The model under review builds one solid part; all positions refer to its coordinate system, in mm. A direction names the side the tool comes from. Coordinates: 2 decimals unless noted, no trailing zeros. Loops run counter-clockwise (first coordinate to the right, second up) from the corner with the lowest first, then second, coordinate; pieces in that order, holes last. Notation, with made-up numbers: M -12,14 L 3,14 A21 ccw 3,45 Z; hole C 39.5,-0.5 d11. An arc over 180 degrees is marked long. One line per item, written item: value.
```python
from build123d import *

# Parameters (mm, degrees)
ESQUISSE1_R        = 6
ESQUISSE1_R_2      = 4
BOSS_EXTRU_1_DEPTH = 17.5
CONG_2_R           = 2
CONG_3_R           = 1
CONG_4_R           = 1


with BuildPart() as part:
    # Esquisse1 → Boss.-Extru.1 (new body)
    # profile 1 of 2: a face of its own
    with BuildSketch(Plane.XY):
        Circle(ESQUISSE1_R)
        Circle(ESQUISSE1_R_2, mode=Mode.SUBTRACT)
    # profile 2 of 2: a face of its own
    with BuildSketch(Plane.XY):
        with BuildLine():
            Line((23.543392678, 29), (-3.675906783, 4.742120762))
            ThreePointArc((-3.675906783, 4.742120762), (2.640507461, 5.387737962), (6, 0))
            ThreePointArc((6, 0), (4.242640687, -4.242640687), (0, -6))
            Line((0, -6), (60, -6))
            Line((60, -6), (60, 0))
            Line((60, 0), (23.543392678, 0))
            Line((23.543392678, 0), (23.543392678, 29))
        make_face()
    extrude(amount=-BOSS_EXTRU_1_DEPTH)

    # Congé2
    cong_2_edges = [part.edges().sort_by_distance(p)[0] for p in [
        (23.543392678, 29, -8.75),
    ]]
    fillet(cong_2_edges, radius=CONG_2_R)

    # Congé3
    cong_3_edges = [part.edges().sort_by_distance(p)[0] for p in [
        (60, 0, -8.75),
    ]]
    fillet(cong_3_edges, radius=CONG_3_R)

    # Congé4
    cong_4_edges = [part.edges().sort_by_distance(p)[0] for p in [
        (60, -6, -8.75),
    ]]
    fillet(cong_4_edges, radius=CONG_4_R)


solid = part.part
```
(1) Tool access review of faces 1 (the face through (60, -3, -9)), 2 (the face through (42, 0, -9)): name each direction out of +Z, -Z, +X, -X, +Y, -Y from which nothing blocks a thin tool from reaching the whole face with its end or side.
Checks:
face 1: +Z, -Z, +X, +Y, -Y
face 2: +Z, -Z, +X, +Y
(2) To check wall thickness, follow L1, parallel to Y at x = 40.5, z = -12.25; L2, parallel to Y at x = 0, z = -7.25; L3, parallel to X at y = 10.5, z = -5.75. State the ranges of each line that lie inside material, in increasing order. Write a range as [from, to].
Checks:
L1: [-6, 0]
L2: [-6, -4], [4, 8.02]
L3: [2.78, 23.54]
(3) Insertion check: pin 1 Ø3 at (y, z) = (1, -10.5) entering from +X; pin 2 Ø3 at (y, z) = (2.5, -11.5) entering from +X; pin 3 Ø3 at (y, z) = (0.5, -10) entering from +X; pin 4 Ø5 at (x, z) = (48, -13) entering from +Y. Each pin has a flat end and moves straight along its axis. Give the tip position at first contact, or say it passes through.
Checks:
pin 1: x = 59.87
pin 2: x = 23.54
pin 3: x = 60
pin 4: y = 0
(4) Draft analysis for pull direction Y (two halves, no side actions). For faces 3 (the face through (-0.867, -3.905, -8.628)), 4 (the face through (-5.71, -1.84, -8.63)), 5 (the face through (8.44, 15.54, -8.63)), state which applies: pulls with the +Y half, pulls with the -Y half, needs draft (parallel to the pull), parting line crosses it, or undercut.
Checks:
face 3: undercut
face 4: parting line crosses it
face 5: pulls with the +Y half
(5) Add section C-C on y = 9.5. State the section outline as (x, z) points, then the cut area to 3 significant figures.
Checks:
outline: M 1.66,-17.5 L 23.54,-17.5 L 23.54,0 L 1.66,0 Z
area: 383 mm^2
(6) Add section B-B on x = 32. State the section outline as (y, z) points.
Checks:
outline: M -6,-17.5 L 0,-17.5 L 0,0 L -6,0 Z
(7) Add section A-A on z = -13. State the section outline as (x, y) points.
Checks:
outline: M -3.68,4.74 A6 ccw 0,-6 L 59,-6 A1 ccw 60,-5 L 60,-1 A1 ccw 59,0 L 23.54,0 L 23.54,24.54 A2 ccw 20.21,26.03 Z; hole C 0,0 d8
